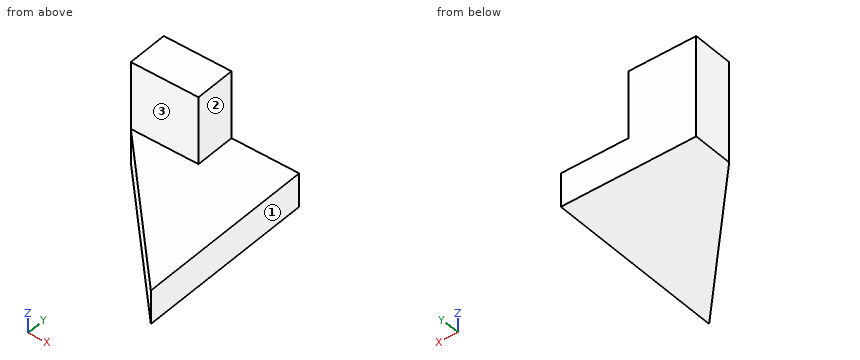
from build123d import *

# Parameters (mm, degrees)
BOSS_EXTRUDE1_DEPTH = 10
SKETCH1_4_W         = 20
SKETCH1_4_H         = 12
BOSS_EXTRUDE2_DEPTH = 30


with BuildPart() as part:
    # Sketch1 → Boss-Extrude1 (new body)
    with BuildSketch(Plane.XY):
        Polygon((20, -12), (0, -12), (40, -54), (40, 0), (20, 0), align=None)
    extrude(amount=BOSS_EXTRUDE1_DEPTH)

    # Sketch1<4> → Boss-Extrude2 (add)
    with BuildSketch(Plane.XY):
        with Locations((10, -6)):
            Rectangle(SKETCH1_4_W, SKETCH1_4_H)
    extrude(amount=BOSS_EXTRUDE2_DEPTH)


solid = part.part
Verification items for the finished model (mm, model axes). Face numbers are marked on the shaded views. A direction names the side the tool comes from. Coordinates: 2 decimals unless noted, no trailing zeros. Loops run counter-clockwise (first coordinate to the right, second up) from the corner with the lowest first, then second, coordinate; pieces in that order, holes last. Notation, with made-up numbers: (26, -31.75) -> (55, -31.75) arc R21 cw to (55, -22.75) -> close; hole circle Ø6 at (70.25, -25). An arc over 180 degrees is marked (long way). Answer as a JSON object with one key per item and string values. Group by question number.
Item 1: Sectioned sample at D-D on x = 31.5. Record the boundary of the cut face in (y, z) (3 decimals).
Item 2: Sectioned sample at A-A on x = 3. Record the boundary of the cut face in (y, z).
Item 3: Scan lines: probe 1 along Y at (x, z) = (16, 28.5); probe 2 along X at (y, z) = (-7, 26.5); probe 3 along Z at (x, y) = (26, -34.5). Record each from-to range of solid material in increasing order.
Item 4: Sectioned sample at C-C on y = -9. Record the boundary of the cut face in (x, z).
Item 5: Sectioned sample at B-B on z = 17. Record the boundary of the cut face in (x, y).
Item 6: Tool access check on the marked faces 1, 2 and 3. Record the directions out of +Z, -Z, +X, -X, +Y, -Y that give a thin tool (end or side, any length) a straight path to the whole face; none if there is none.
Item 7: Depth check by flat-ended pin: pin 1 (5 mm diameter, centred on x = 9.5, z = 5.5, fed in from +Y); pin 2 (20 mm diameter, centred on x = 28.5, y = -17.5, fed in from +Z); pin 3 (10 mm diameter, centred on x = 8, z = 19.5, fed in from -Y). Enter the tip coordinate at first touch or a pass-through.
Evaluation:
{
 "1": {"outline": "(-45.075, 0) -> (0, 0) -> (0, 10) -> (-45.075, 10) -> close"},
 "2": {"outline": "(-15.15, 0) -> (0, 0) -> (0, 30) -> (-12, 30) -> (-12, 10) -> (-15.15, 10) -> close"},
 "3": {"probe 1": "y = -12 to 0", "probe 2": "x = 0 to 20", "probe 3": "z = 0 to 10"},
 "4": {"outline": "(0, 0) -> (40, 0) -> (40, 10) -> (20, 10) -> (20, 30) -> (0, 30) -> close"},
 "5": {"outline": "(0, -12) -> (20, -12) -> (20, 0) -> (0, 0) -> close"},
 "6": {"face 1": "+Z, -Z, +X, +Y, -Y", "face 2": "+Z, +X, +Y, -Y", "face 3": "+Z, +X, -X, -Y"},
 "7": {"pin 1": "stops at y = 0", "pin 2": "stops at z = 10", "pin 3": "stops at y = -12"}
}
